The listing builds one solid part. Answer for the finished solid, in the listing's coordinates (mm). A direction names the side the tool comes from. Give positions to 0.01 mm unless a question says otherwise; leave off trailing zeros. Loops run counter-clockwise (first coordinate to the right, second up) from the corner with the lowest first, then second, coordinate; pieces in that order, holes last. Notation, with made-up numbers: (56.5, 29) - (109.5, 29) arc R15 cw to (109.5, 38) - close; hole circle Ø7 at (32, -19). An arc over 180 degrees is marked (long way). Write each question's results on one line, items separated by ' | '.
from build123d import *

# Parameters (mm, degrees)
SKETCH1_R                 = 7
BOSS_EXTRUDE1_DEPTH       = 21
SKETCH3_W                 = 3
SKETCH3_H                 = 3
CUT_EXTRUDE1_DEPTH        = 21
SKETCH6_R                 = 8.5
BOSS_EXTRUDE2_DEPTH       = 24
SKETCH7_R                 = 10
BOSS_EXTRUDE3_DEPTH       = 17
FILLET1_R                 = 0.6
SKETCH8_R                 = 11.25
BOSS_EXTRUDE4_DEPTH       = 2
SKETCH10_R                = 11
SKETCH10_W                = 10
SKETCH10_H                = 10
CUT_EXTRUDE2_DEPTH        = 5
M4X0_7_TAPPED_HOLE1_D     = 3.3
M4X0_7_TAPPED_HOLE1_DEPTH = 20
M4X0_7_TAPPED_HOLE1_TIP   = 0.991420021


with BuildPart() as part:
    # Sketch1 → Boss-Extrude1 (new body)
    with BuildSketch(Plane.XY):
        Circle(SKETCH1_R)
    extrude(amount=BOSS_EXTRUDE1_DEPTH)

    # Sketch3 → Cut-Extrude1 (cut)
    with BuildSketch(Plane(origin=(0, 0, 0), x_dir=(-1, 0, 0), z_dir=(0, 0, -1))):
        with Locations((0, 7)):
            Rectangle(SKETCH3_W, SKETCH3_H)
    extrude(amount=-CUT_EXTRUDE1_DEPTH, mode=Mode.SUBTRACT)

    # Sketch6 → Boss-Extrude2 (add)
    with BuildSketch(Plane.XY.offset(21)):
        Circle(SKETCH6_R)
    extrude(amount=BOSS_EXTRUDE2_DEPTH)

    # Sketch7 → Boss-Extrude3 (add)
    with BuildSketch(Plane.XY.offset(45)):
        Circle(SKETCH7_R)
    extrude(amount=BOSS_EXTRUDE3_DEPTH)

    # Fillet1
    fillet1_edges = [part.edges().sort_by_distance(p)[0] for p in [
        (-8.5, 0, 45),
    ]]
    fillet(fillet1_edges, radius=FILLET1_R)

    # Sketch8 → Boss-Extrude4 (add)
    with BuildSketch(Plane(origin=(0, 0, 45), x_dir=(-1, 0, 0), z_dir=(0, 0, -1))):
        Circle(SKETCH8_R)
    extrude(amount=-BOSS_EXTRUDE4_DEPTH)

    # Sketch10 → Cut-Extrude2 (cut)
    with BuildSketch(Plane.XY.offset(57)):
        Circle(SKETCH10_R)
        Rectangle(SKETCH10_W, SKETCH10_H, mode=Mode.SUBTRACT)
    extrude(amount=CUT_EXTRUDE2_DEPTH, mode=Mode.SUBTRACT)

    # M4x0.7 Tapped Hole1
    with Locations(Plane.XY.offset(62)):
        with Locations((0, 0)):
            Hole(M4X0_7_TAPPED_HOLE1_D / 2, depth=M4X0_7_TAPPED_HOLE1_DEPTH)
            with Locations((0, 0, -(M4X0_7_TAPPED_HOLE1_DEPTH + M4X0_7_TAPPED_HOLE1_TIP / 2))):  # 118° drill point
                Cone(0, M4X0_7_TAPPED_HOLE1_D / 2, M4X0_7_TAPPED_HOLE1_TIP, mode=Mode.SUBTRACT)


solid = part.part
Item 1: Flat-ended cylindrical pins translate along their axes: P1, Ø5.5, axis at y = -0.5, z = 59.5, coming from the +X side; P2, Ø2.5, axis at x = 0, y = 0, coming from the +Z side; P3, Ø1.5, axis at x = 1, z = 59.5, coming from the -Y side. Find the tip coordinate at first contact, or state that the pin passes through.
Values found:
P1: stops at x = 10 | P2: stops at z = 41.76 | P3: stops at y = -5
Item 2: For a pull along Y with two mould halves and no side action, classify faces 4 (the face through (-0.1, -0.3, 41.2)), 5 (the face through (0, -7, 10)), 6 (the face through (0, -5, 59)), 7 (the face through (5, 0, 59)) as released by +Y, released by -Y, zero draft, split by the parting line, or undercut.
Values found:
face 4: undercut | face 5: split by the parting line | face 6: released by -Y | face 7: zero draft
Item 3: For faces 1 (the face through (-5, 0, 59)), 2 (the face through (-1.5, 6, 10)), 3 (the face through (0, 5, 59)), determine the directions among +Z, -Z, +X, -X, +Y, -Y from which every point of the face is accessible in a straight line to the end or side of a thin tool.
Values found:
face 1: +Z, -X, +Y, -Y | face 2: -Z, +Y | face 3: +Z, +X, -X, +Y
Item 4: A cutting plane is placed at A-A, the plane z = 25. Determine the outline of the cut face in (x, y), plus the area to 3 significant figures.
Values found:
outline: circle Ø17 at (0, 0) | area: 227 mm²
Item 5: Find the intervals of material crossed by line 1 along X through (y, z) = (0, 55.75); line 2 along X through (y, z) = (0, 57.75); line 3 along Z through (x, y) = (7, -1), in increasing order. Write a range as [from, to].
Values found:
line 1: x = [-10, -1.65], [1.65, 10] | line 2: x = [-5, -1.65], [1.65, 5] | line 3: z = [21, 57]
